For this review, use the dimensioned drawing (mm, ordinates from the lowest corner) and the shaded views. Coordinates: 2 decimals unless noted, no trailing zeros. Loops run counter-clockwise (first coordinate to the right, second up) from the corner with the lowest first, then second, coordinate; pieces in that order, holes last.
1. Clearance check with a flat-ended pin moving along its axis: P1, Ø1.5, axis at x = 33.5, y = 5, coming from the -Z side. State where the tip first meets the part, or that it passes through.
2. To check wall thickness, follow probe 1 along X at (y, z) = (5.25, 10.5); probe 2 along X at (y, z) = (5, 2.54); probe 3 along Z at (x, y) = (27.5, 0.5). State the ranges of each line that lie inside material, in increasing order.
3. Take a section at A-A, the plane z = 48.26. State the section outline as (x, y) points.
4. Take a section at B-B, the plane y = 2.5. Count the separate pieces of the cut face and the enclosed holes in it, then the cut area to 3 significant figures.
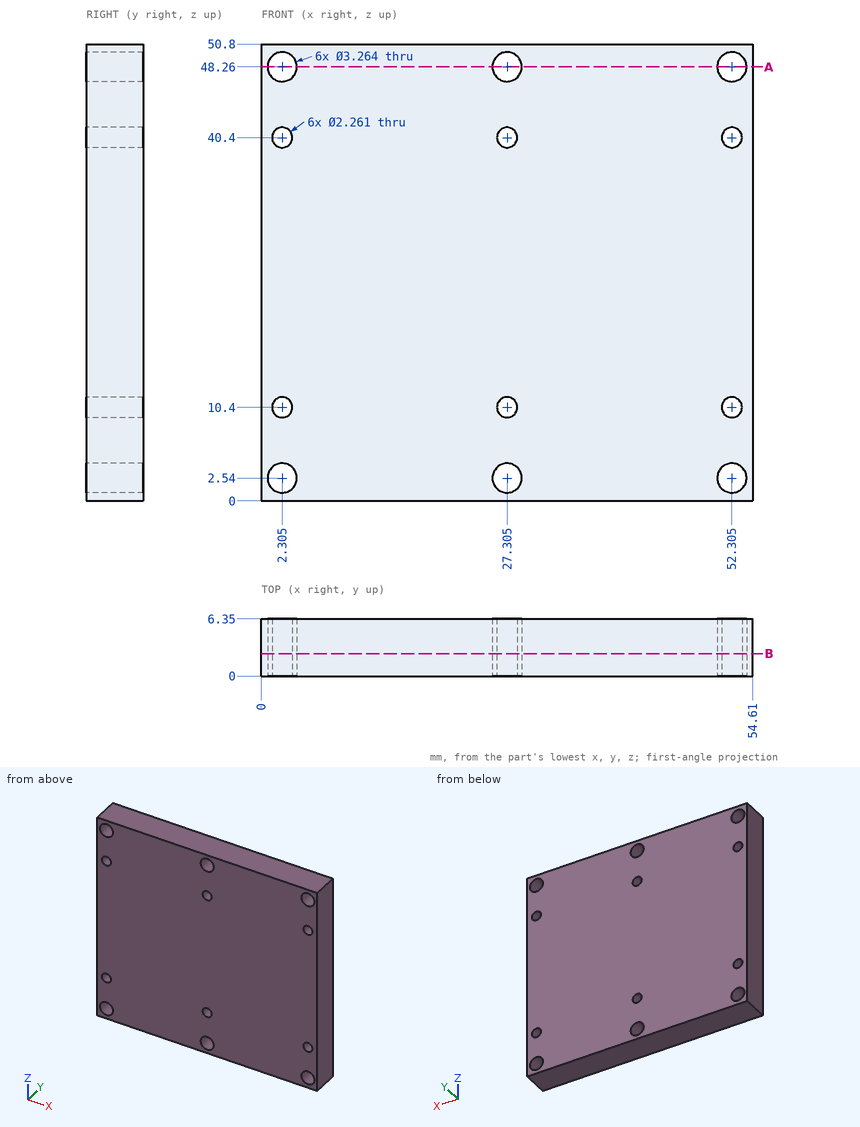
Results list:
1. P1: stops at z = 0
2. probe 1: x = 0 to 1.18, 3.43 to 26.18, 28.43 to 51.18, 53.43 to 54.61
2. probe 2: x = 0 to 0.67, 3.94 to 25.67, 28.94 to 50.67, 53.94 to 54.61
2. probe 3: z = 0 to 0.92, 4.16 to 9.29, 11.51 to 39.29, 41.51 to 46.64, 49.88 to 50.8
3. outline: (0, 0) - (0.67, 0) - (0.67, 6.35) - (0, 6.35) - close; (3.94, 0) - (25.67, 0) - (25.67, 6.35) - (3.94, 6.35) - close; (28.94, 0) - (50.67, 0) - (50.67, 6.35) - (28.94, 6.35) - close; (53.94, 0) - (54.61, 0) - (54.61, 6.35) - (53.94, 6.35) - close
4. separate pieces: 1
4. enclosed holes: 12
4. area: 2,700 mm2
